Model file for the job. Use its own axes, mm. Face numbers are marked on the shaded views. A direction names the side the tool comes from. Round coordinates to 2 decimals unless told otherwise and drop trailing zeros. Loops run counter-clockwise (first coordinate to the right, second up) from the corner with the lowest first, then second, coordinate; pieces in that order, holes last. Notation, with made-up numbers: (-32, -5.75) - (1, -5.75) arc R27 ccw to (1, 24.25) - close; hole circle Ø1 at (-6.5, 58). An arc over 180 degrees is marked (long way). Answer as a JSON object with one key per item and string values.
from build123d import *

# Parameters (mm, degrees)
F1_DEPTH = 12.7
F2_DEPTH = 17.78


with BuildPart() as f1:
    # F0 (on Front) → F1 (new body)
    with BuildSketch(Plane.XZ):
        with BuildLine():
            ThreePointArc((-7.62, 24.2300557169), (-3.8546455617, 25.1058102362), (0, 25.4))
            Line((0, 25.4), (0, 31.7809050116))
            ThreePointArc((0, 31.7809050116), (-1.3343592112, 31.7528803237), (-2.6663651224, 31.6688556849))
            Line((-2.6663651224, 31.6688556849), (-2.6663651224, 29.21))
            Line((-2.6663651224, 29.21), (-4.8713176511, 29.21))
            Line((-4.8713176511, 29.21), (-4.8713176511, 31.405352851))
            ThreePointArc((-4.8713176511, 31.405352851), (-6.251742675, 31.1599364069), (-7.62, 30.8538737172))
            Line((-7.62, 30.8538737172), (-7.62, 24.2300557169))
        make_face()
        with BuildLine():
            ThreePointArc((-7.62, -24.2300557169), (-25.400000003, 0), (-7.62, 24.2300557169))
            Line((-7.62, 24.2300557169), (-7.62, 30.8538737172))
            ThreePointArc((-7.62, 30.8538737172), (-31.7809050116, 0), (-7.62, -30.8538737172))
            Line((-7.62, -30.8538737172), (-7.62, -24.2300557169))
        make_face()
        with BuildLine():
            ThreePointArc((-2.6663651224, 31.6688556849), (-1.3343592112, 31.7528803237), (0, 31.7809050116))
            Line((0, 31.7809050116), (0, 39.37))
            Line((0, 39.37), (-7.62, 39.37))
            Line((-7.62, 39.37), (-7.62, 30.8538737172))
            ThreePointArc((-7.62, 30.8538737172), (-6.251742675, 31.1599364069), (-4.8713176511, 31.405352851))
            Line((-4.8713176511, 31.405352851), (-4.8713176511, 36.0698501384))
            Line((-4.8713176511, 36.0698501384), (-2.6663651224, 36.0698501384))
            Line((-2.6663651224, 36.0698501384), (-2.6663651224, 31.6688556849))
        make_face()
        with BuildLine():
            ThreePointArc((0, -25.4), (-3.8546455617, -25.1058102362), (-7.62, -24.2300557169))
            Line((-7.62, -24.2300557169), (-7.62, -30.8538737172))
            ThreePointArc((-7.62, -30.8538737172), (-6.251742675, -31.1599364069), (-4.8713176511, -31.405352851))
            Line((-4.8713176511, -31.405352851), (-4.8713176511, -29.21))
            Line((-4.8713176511, -29.21), (-2.6663651224, -29.21))
            Line((-2.6663651224, -29.21), (-2.6663651224, -31.6688556849))
            ThreePointArc((-2.6663651224, -31.6688556849), (-1.3343592112, -31.7528803237), (0, -31.7809050116))
            Line((0, -31.7809050116), (0, -25.4))
        make_face()
        with BuildLine():
            ThreePointArc((-4.8713176511, -31.405352851), (-6.251742675, -31.1599364069), (-7.62, -30.8538737172))
            Line((-7.62, -30.8538737172), (-7.62, -39.37))
            Line((-7.62, -39.37), (0, -39.37))
            Line((0, -39.37), (0, -31.7809050116))
            ThreePointArc((0, -31.7809050116), (-1.3343592112, -31.7528803237), (-2.6663651224, -31.6688556849))
            Line((-2.6663651224, -31.6688556849), (-2.6663651224, -36.0698501384))
            Line((-2.6663651224, -36.0698501384), (-4.8713176511, -36.0698501384))
            Line((-4.8713176511, -36.0698501384), (-4.8713176511, -31.405352851))
        make_face()
    extrude(amount=F1_DEPTH)

    # F0 (on Front) → F2 (join)
    with BuildSketch(Plane.XZ):
        with BuildLine():
            ThreePointArc((-7.62, -24.2300557169), (-25.400000003, 0), (-7.62, 24.2300557169))
            Line((-7.62, 24.2300557169), (-7.62, 30.8538737172))
            ThreePointArc((-7.62, 30.8538737172), (-31.7809050116, 0), (-7.62, -30.8538737172))
            Line((-7.62, -30.8538737172), (-7.62, -24.2300557169))
        make_face()
    extrude(amount=F2_DEPTH)


solid = f1.part
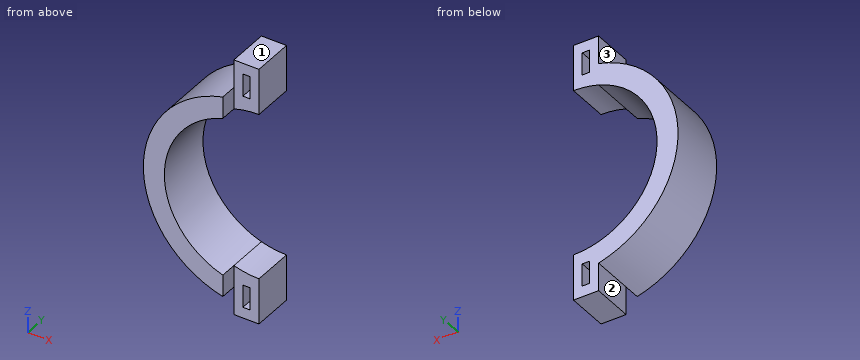
1) Slice it at D-D on y = -13.75. List the corners of the cut face in (x, z), then the cut area to 3 significant figures.
Values follow:
{"outline": "(-7.62, -30.85) - (-7.62, -24.23) arc R25.4 cw to (-7.62, 24.23) - (-7.62, 30.85) arc R31.78 ccw to start", "area": "475 mm²"}
2) Slice it at B-B on x = -10. List the corners of the cut face in (y, z).
Values follow:
{"outline": "(-17.78, -30.17) - (0, -30.17) - (0, -23.35) - (-17.78, -23.35) - close; (-17.78, 23.35) - (0, 23.35) - (0, 30.17) - (-17.78, 30.17) - close"}
3) Slice it at A-A on z = -34. List the corners of the cut face in (x, y), then the cut area to 3 significant figures.
Values follow:
{"outline": "(-7.62, -12.7) - (-4.87, -12.7) - (-4.87, 0) - (-7.62, 0) - close; (-2.67, -12.7) - (0, -12.7) - (0, 0) - (-2.67, 0) - close", "area": "68.8 mm²"}
4) Probe probe 1 along X at (y, z) = (-9.5, 32); probe 2 along Z at (x, y) = (-4, -5); probe 3 along Z at (x, y) = (-1.5, -1.75). List the from-to ranges inside material, lowest first.
Values follow:
{"probe 1": "-7.62 to -4.87, -2.67 to 0", "probe 2": "-39.37 to -36.07, -29.21 to -25.08, 25.08 to 29.21, 36.07 to 39.37", "probe 3": "-39.37 to -25.36, 25.36 to 39.37"}
5) Tool access for the marked faces 1, 2 and 3: list every direction of +Z, -Z, +X, -X, +Y, -Y with a clear straight run to the whole face (end or side of a thin tool).
Values follow:
{"face 1": "+Z, +X, -X, +Y, -Y", "face 2": "-Z, -X, +Y, -Y", "face 3": "+Z, -X, +Y, -Y"}
6) Slice it at C-C on y = -9.75. List the corners of the cut face in (x, z), then the cut area to 3 significant figures.
Values follow:
{"outline": "(-7.62, -39.37) - (0, -39.37) - (0, -25.4) arc R25.4 cw to (0, 25.4) - (0, 39.37) - (-7.62, 39.37) - (-7.62, 30.85) arc R31.78 ccw to (-7.62, -30.85) - close; hole (-4.87, -36.07) - (-2.67, -36.07) - (-2.67, -29.21) - (-4.87, -29.21) - close; hole (-4.87, 29.21) - (-2.67, 29.21) - (-2.67, 36.07) - (-4.87, 36.07) - close", "area": "663 mm²"}
7) Drop flat-ended pins along their axis: P1, Ø4.5, axis at y = -8.5, z = -35.5, coming from the -X side; P2, Ø2.5, axis at x = -2.5, z = -31.5, coming from the -Y side; P3, Ø5.5, axis at y = -6.5, z = -31, coming from the -X side. Give the stop position or say it passes through.
Values follow:
{"P1": "x = -7.62", "P2": "y = -12.7", "P3": "x = -14.56"}
